from build123d import *

# Parameters (mm, degrees)
F0_W     = 76.2
F0_H     = 38.1
F1_DEPTH = 5.08
F2_W     = 31.75
F2_H     = 10.16
F3_DEPTH = 5.08
F4_R     = 1.905
F5_DEPTH = 5.08
F7_DEPTH = 2.54
F8_R     = 5.08


with BuildPart() as f1:
    # F0 (on Top) → F1 (new body)
    with BuildSketch(Plane.XY):
        Rectangle(F0_W, F0_H)
    extrude(amount=F1_DEPTH)

    # F2 (on face) → F3 (cut, through all)
    with BuildSketch(Plane.XY.offset(5.08)):
        Rectangle(F2_W, F2_H)
    extrude(amount=-F3_DEPTH, mode=Mode.SUBTRACT)

    # F4 (on face) → F5 (cut, through all)
    with BuildSketch(Plane.XY.offset(5.08)):
        with Locations((-22.225, 0)):
            Circle(F4_R)
        with BuildLine():
            ThreePointArc((24.13, 0), (22.225, 1.905), (20.32, 0))
            ThreePointArc((20.32, 0), (22.225, -1.905), (24.13, 0))
        make_face()
    extrude(amount=-F5_DEPTH, mode=Mode.SUBTRACT)

    # F6 (on face) → F7 (cut)
    with BuildSketch(Plane.XY.offset(5.08)):
        Polygon((-18.669, 0), (-20.447, 3.079586), (-24.003, 3.079586), (-25.781, 0), (-24.003, -3.079586), (-20.447, -3.079586), align=None)
        Polygon((25.781, 0), (24.003, 3.079586), (20.447, 3.079586), (18.669, 0), (20.447, -3.079586), (24.003, -3.079586), align=None)
    extrude(amount=-F7_DEPTH, mode=Mode.SUBTRACT)

    # F8
    f8_edges = [f1.edges().sort_by_distance(p)[0] for p in [
        (38.1, -19.05, 2.54),
        (38.1, 19.05, 2.54),
        (-38.1, 19.05, 2.54),
        (-38.1, -19.05, 2.54),
    ]]
    fillet(f8_edges, radius=F8_R)


solid = f1.part
Design review of the part built by this model. Coordinates are the model's own, in mm. A direction names the side the tool comes from. Round coordinates to 2 decimals unless told otherwise and drop trailing zeros. Write each loop counter-clockwise with the first axis right and the second up, starting at its lowest first coordinate (ties: lowest second). Pieces come first, ordered by that corner, then holes.
Item 1: Draft analysis for pull direction X (two halves, no side actions). For faces 1 (the flat face through (-24.904, -1.518, 3.828)), 2 (the flat face through (24.88, -1.56, 3.83)), 3 (the cylindrical face through (36.572, 17.601, 2.576)), 4 (the flat face through (0, -19.05, 3)), state which applies: released by +X, released by -X, zero draft, split by the parting line, or undercut.
Item 2: For faces 5 (the flat face through (0, -5.08, 3)), 6 (the flat face through (22, -3.08, 4)), 7 (the cylindrical face through (-36.651, -17.522, 2.576)), list the 3-axis set-ups (+Z, -Z, +X, -X, +Y, -Y) from which the entire face can be reached by the end or side of a thin tool; tool diameter is ignored.
Item 3: Consider section A-A on z = 3.55. Give the boundary of the cut face in (x, y) (3 decimals).
Item 4: Consider section B-B on x = -22.5. Give the boundary of the cut face in (y, z).
Item 5: For pin 1 Ø12 at (x, y) = (21.5, 6) entering from -Z; pin 2 Ø5 at (x, y) = (22.225, 0) entering from +Z; pin 3 Ø1.8 at (x, y) = (-22, -0.5) entering from +Z, all flat-tipped, find the tip position at first contact; note any pin that passes through.
Item 6: Wall thickness on L1, parallel to Y at x = 9, z = 1.15; L2, parallel to X at y = -3.5, z = 1.6 (3 decimals); L3, parallel to X at y = -1, z = 0.6 (3 decimals): over which ranges is each line inside the solid? List them lowest first.
Check values:
1. face 1: undercut
1. face 2: undercut
1. face 3: released by +X
1. face 4: zero draft
2. face 5: +Z, -Z
2. face 6: +Z
2. face 7: +Z, -Z, -X, -Y
3. outline: (-38.1, -13.97) arc R5.08 ccw to (-33.02, -19.05) - (33.02, -19.05) arc R5.08 ccw to (38.1, -13.97) - (38.1, 13.97) arc R5.08 ccw to (33.02, 19.05) - (-33.02, 19.05) arc R5.08 ccw to (-38.1, 13.97) - close; hole (-25.781, 0) - (-24.003, -3.08) - (-20.447, -3.08) - (-18.669, 0) - (-20.447, 3.08) - (-24.003, 3.08) - close; hole (-15.875, -5.08) - (15.875, -5.08) - (15.875, 5.08) - (-15.875, 5.08) - close; hole (18.669, 0) - (20.447, -3.08) - (24.003, -3.08) - (25.781, 0) - (24.003, 3.08) - (20.447, 3.08) - close
4. outline: (-19.05, 0) - (-1.89, 0) - (-1.89, 2.54) - (-3.08, 2.54) - (-3.08, 5.08) - (-19.05, 5.08) - close; (1.89, 0) - (19.05, 0) - (19.05, 5.08) - (3.08, 5.08) - (3.08, 2.54) - (1.89, 2.54) - close
5. pin 1: stops at z = 0
5. pin 2: stops at z = 2.54
5. pin 3: passes through
6. L1: y = -19.05 to -5.08, 5.08 to 19.05
6. L2: x = -38.1 to -15.875, 15.875 to 38.1
6. L3: x = -38.1 to -23.846, -20.604 to -15.875, 15.875 to 20.604, 23.846 to 38.1
